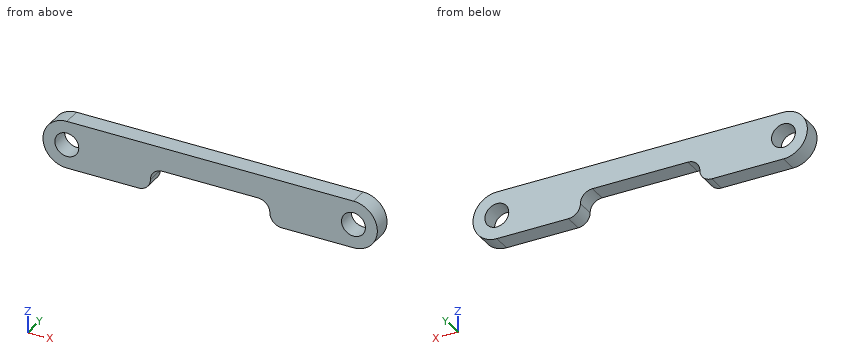
```python
from build123d import *

# Parameters (mm, degrees)
SKETCH1_R           = 1.27
BOSS_EXTRUDE1_DEPTH = 1.905
FILLET1_START       = -1
FILLET1_DEPTH       = 4
FILLET1_2_DEPTH     = 1.905


with BuildPart() as part:
    # Sketch1 → Boss-Extrude1 (new body)
    with BuildSketch(Plane(origin=(0, 0, 0), x_dir=(1, 0, 0), z_dir=(0, 1, 0))):
        with BuildLine():
            Line((6.35, 2.54), (6.35, 0))
            Line((6.35, 0), (-6.35, 0))
            Line((-6.35, 0), (-6.35, 2.54))
            Line((-6.35, 2.54), (-15.24, 2.54))
            ThreePointArc((-15.24, 2.54), (-17.78, 0), (-15.24, -2.54))
            Line((-15.24, -2.54), (15.24, -2.54))
            ThreePointArc((15.24, -2.54), (17.78, 0), (15.24, 2.54))
            Line((15.24, 2.54), (6.35, 2.54))
        make_face()
        with Locations(Location((-15.24, 0, 0), (0, 0, 90))):
            Circle(SKETCH1_R, mode=Mode.SUBTRACT)
        with Locations(Location((15.24, 0, 0), (0, 0, 90))):
            Circle(SKETCH1_R, mode=Mode.SUBTRACT)
    extrude(amount=BOSS_EXTRUDE1_DEPTH)

    # Fillet1: read off the stored shape, not the designer's step
    # Fillet1 outline → Fillet1 (cut)
    with BuildSketch(Plane(origin=(0, 0, 0), x_dir=(1, 0, 0), z_dir=(0, 1, 0)).offset(FILLET1_START)):
        with BuildLine():
            Line((6.35, 2.54), (6.35, 1.27))
            ThreePointArc((6.35, 1.27), (6.721974388, 2.168025612), (7.62, 2.54))
            Line((7.62, 2.54), (6.35, 2.54))
        make_face()
        with BuildLine():
            ThreePointArc((-7.62, 2.54), (-6.721974388, 2.168025612), (-6.35, 1.27))
            Line((-6.35, 1.27), (-6.35, 2.54))
            Line((-6.35, 2.54), (-7.62, 2.54))
        make_face()
    extrude(amount=FILLET1_DEPTH, mode=Mode.SUBTRACT)

    # Fillet1 2 outline → Fillet1 2 (add)
    with BuildSketch(Plane(origin=(0, 0, 0), x_dir=(1, 0, 0), z_dir=(0, 1, 0))):
        with BuildLine():
            Line((-6.35, 0), (-5.08, 0))
            ThreePointArc((-5.08, 0), (-5.978025612, 0.371974388), (-6.35, 1.27))
            Line((-6.35, 1.27), (-6.35, 0))
        make_face()
        with BuildLine():
            ThreePointArc((6.35, 1.27), (5.978025612, 0.371974388), (5.08, 0))
            Line((5.08, 0), (6.35, 0))
            Line((6.35, 0), (6.35, 1.27))
        make_face()
    extrude(amount=FILLET1_2_DEPTH)


solid = part.part
```
The listing builds one solid part. Answer for the finished solid, in the listing's coordinates (mm). Coordinates: 2 decimals unless noted, no trailing zeros. Order: outer loops, then holes, each group sorted by start corner. A loop starts at its lowest first (then second) coordinate and runs counter-clockwise, first axis right, second up. Notation, with made-up numbers: M -9.5,-10 L 18.5,-10 A27 cw 18.5,13 Z; hole C -21.75,44.5 d8. An arc over 180 degrees is marked long. Answer as a JSON object with one key per item and string values. Group by question number.
1. Straight lines are drawn through the part: line 1 (X direction, y = 0.4, z = -0.2); line 2 (X direction, y = 1.1, z = 1); line 3 (Z direction, x = 15.24, y = 0.5). For each, find the intervals that lie inside material, in ascending order.
2. Flat-ended cylindrical pins translate along their axes: P1, Ø1, axis at y = 1.5, z = 2, coming from the +X side; P2, Ø0.6, axis at x = -0.5, y = 0.5, coming from the -Z side; P3, Ø3, axis at x = 15.24, z = 0, coming from the -Y side. Find the tip coordinate at first contact, or state that the pin passes through.
3. Section B-B on z = -1.95 is taken. Write down the section's boundary in (x, y) (3 decimals).
4. Section C-C on x = -7 is taken. Write down the section's boundary in (y, z) (3 decimals).
5. Section A-A on y = 0.45 is taken. Write down the section's boundary in (x, z), then the cut area to 3 significant figures.
Values follow:
{
 "1": {"line 1": "-17.77 to -16.49, -13.99 to -5.76, 5.76 to 13.99, 16.49 to 17.77", "line 2": "-17.57 to -16.02, -14.46 to 14.46, 16.02 to 17.57", "line 3": "-2.54 to -1.27, 1.27 to 2.54"},
 "2": {"P1": "x = 17.29", "P2": "z = 0", "P3": "y = 0"},
 "3": {"outline": "M -16.868,0 L -6.547,0 L -6.547,1.905 L -16.868,1.905 Z; M 6.547,0 L 16.868,0 L 16.868,1.905 L 6.547,1.905 Z"},
 "4": {"outline": "M 0,-2.378 L 1.905,-2.378 L 1.905,2.54 L 0,2.54 Z"},
 "5": {"outline": "M -15.24,-2.54 L -7.62,-2.54 A1.27 ccw -6.35,-1.27 A1.27 cw -5.08,0 L 5.08,0 A1.27 cw 6.35,-1.27 A1.27 ccw 7.62,-2.54 L 15.24,-2.54 A2.54 ccw 15.24,2.54 L -15.24,2.54 A2.54 ccw Z; hole C -15.24,0 d2.54; hole C 15.24,0 d2.54", "area": "133 mm2"}
}
